Check sheet for the drawn part. Datum: minimum x, y, z corner. Units: mm. Round coordinates to 2 decimals unless told otherwise and drop trailing zeros. Write each loop counter-clockwise with the first axis right and the second up, starting at its lowest first coordinate (ties: lowest second). Pieces come first, ordered by that corner, then holes. Notation, with made-up numbers: M 77.25,-7 L 118.25,-7 A20 ccw 118.25,4 Z; hole C 5,76.5 d2. An arc over 180 degrees is marked long. One line per item, written item: value. Start each with the question number.
1. Section check A-A (z = 15). Record the boundary of the cut face in (x, y).
2. Section check C-C (z = 42). Record the boundary of the cut face in (x, y).
3. Depth check by flat-ended pin: P1, Ø5, axis at x = 7, y = 47.5, coming from the -Z side. Enter the tip coordinate at first touch or a pass-through.
4. Section check B-B (y = 17). Record the boundary of the cut face in (x, z).
5. Section check D-D (x = 8.75). Record the boundary of the cut face in (y, z), and give its area (3 significant figures).
6. Scan lines: probe 1 along Z at (x, y) = (4.75, 47); probe 2 along Z at (x, y) = (7.5, 69.75); probe 3 along Y at (x, z) = (6.5, 42). Record each from-to range of solid material in increasing order. Write a range as [from, to].
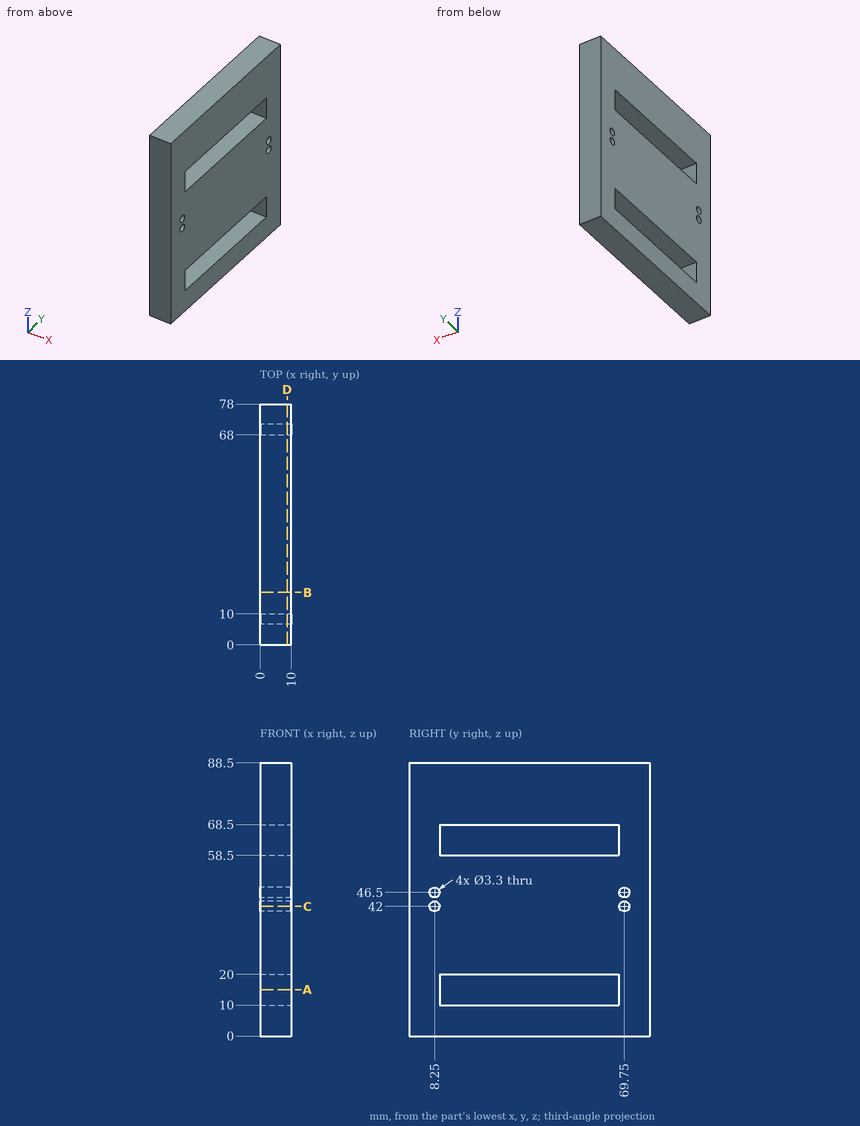
Result sheet:
1. outline: M 0,0 L 10,0 L 10,10 L 0,10 Z; M 0,68 L 10,68 L 10,78 L 0,78 Z
2. outline: M 0,0 L 10,0 L 10,6.6 L 0,6.6 Z; M 0,9.9 L 10,9.9 L 10,68.1 L 0,68.1 Z; M 0,71.4 L 10,71.4 L 10,78 L 0,78 Z
3. P1: stops at z = 0
4. outline: M 0,0 L 10,0 L 10,10 L 0,10 Z; M 0,20 L 10,20 L 10,58.5 L 0,58.5 Z; M 0,68.5 L 10,68.5 L 10,88.5 L 0,88.5 Z
5. outline: M 0,0 L 78,0 L 78,88.5 L 0,88.5 Z; hole C 8.25,42 d3.3; hole C 8.25,46.5 d3.3; hole M 10,10 L 68,10 L 68,20 L 10,20 Z; hole M 10,58.5 L 68,58.5 L 68,68.5 L 10,68.5 Z; hole C 69.75,42 d3.3; hole C 69.75,46.5 d3.3
5. area: 5,710 mm2
6. probe 1: z = [0, 10], [20, 58.5], [68.5, 88.5]
6. probe 2: z = [0, 40.35], [43.65, 44.85], [48.15, 88.5]
6. probe 3: y = [0, 6.6], [9.9, 68.1], [71.4, 78]
